from build123d import *

# Parameters (mm, degrees)
CHAFL_N1_SIZE                       = 1.5
CROQUIS3_W                          = 16
CROQUIS3_H                          = 16
CROQUIS3_R                          = 2
SALIENTE_EXTRUIR1_DEPTH             = 2
SALIENTE_EXTRUIR1_DIRECTION_2_REACH = 43.106


with BuildPart() as part:
    # Croquis1 → Revolución1 (revolve)
    with BuildSketch(Plane.XY, mode=Mode.PRIVATE) as revoluci_n1_sk:
        Polygon((0, 9.55), (24, 9.55), (37.076983597, 2), (37.076983597, 5.464101615), (24.803847577, 12.55), (0, 12.55), align=None)
    revolve(revoluci_n1_sk.sketch.rotate(Axis((0, 0, 0), (1, 0, 0)), 180), axis=Axis((0, 0, 0), (1, 0, 0)))

    # Chaflán1
    chafl_n1_edges = [part.edges().sort_by_distance(p)[0] for p in [
        (0, 9.55, 0),
    ]]
    chamfer(chafl_n1_edges, length=CHAFL_N1_SIZE)

    # Croquis3 → Saliente-Extruir1 (add)
    with BuildSketch(Plane(origin=(37.076983597, 0, 0), x_dir=(0, 0, -1), z_dir=(1, 0, 0))):
        Rectangle(CROQUIS3_W, CROQUIS3_H)
        with Locations(Location((0, 0, 0), (0, 0, 270))):
            Circle(CROQUIS3_R, mode=Mode.SUBTRACT)
    extrude(amount=SALIENTE_EXTRUIR1_DEPTH)

    # Croquis3 → Saliente-Extruir1 direction 2 (add, up to next)
    with BuildSketch(Plane(origin=(37.076983597, 0, 0), x_dir=(0, 0, -1), z_dir=(1, 0, 0)), mode=Mode.PRIVATE) as saliente_extruir1_direction_2_sk1:
        Rectangle(CROQUIS3_W, CROQUIS3_H)
        with Locations(Location((0, 0, 0), (0, 0, 270))):
            Circle(CROQUIS3_R, mode=Mode.SUBTRACT)
    saliente_extruir1_direction_2_tool1 = extrude(saliente_extruir1_direction_2_sk1.sketch, amount=-SALIENTE_EXTRUIR1_DIRECTION_2_REACH, mode=Mode.PRIVATE) - part.part
    add(saliente_extruir1_direction_2_tool1.solids().sort_by_distance((37.076984, -7.773726, 0))[0])


solid = part.part
Geometry check sheet. Reference: the model listing, model coordinates, mm. Give positions to 0.01 mm unless a question says otherwise; leave off trailing zeros. Order: outer loops, then holes, each group sorted by start corner. A loop starts at its lowest first (then second) coordinate and runs counter-clockwise, first axis right, second up. Notation, with made-up numbers: (86.5, 11) - (127.5, 11) arc R22 ccw to (127.5, 41) - close; hole circle Ø2 at (-20, 30.25). An arc over 180 degrees is marked (long way). Answer as a JSON object with one key per item and string values.
(1) Draft check along Y on faces 1 (the cylindrical face through (38, 0, 2)), 2 (the flat face through (34, -8, 0)), 3 (the cylindrical face through (12.91, 7.58, 5.81)), 4 (the conical face through (31.316, -8.12, 3.367)). Enter one of: released by +Y, released by -Y, zero draft, split by the parting line, or undercut.
Report:
{"face 1": "undercut", "face 2": "released by -Y", "face 3": "undercut", "face 4": "split by the parting line"}
(2) Material ranges on line 1 (Z direction, x = 11.25, y = 0); line 2 (Z direction, x = 38.4, y = 0); line 3 (Y direction, x = 14.5, z = 6.25), recorded low to high.
Report:
{"line 1": "-12.55 to -9.55, 9.55 to 12.55", "line 2": "-8 to -2, 2 to 8", "line 3": "-10.88 to -7.22, 7.22 to 10.88"}
(3) Depth check by flat-ended pin: pin 1 Ø4 at (x, y) = (23.5, 6) entering from +Z; pin 2 Ø12 at (x, z) = (9.5, -10) entering from +Y; pin 3 Ø3.5 at (x, y) = (32, 2.5) entering from -Z. Enter the tip coordinate at first touch or a pass-through.
Report:
{"pin 1": "z = 11.9", "pin 2": "y = 11.9", "pin 3": "z = -9.15"}
(4) Cross-section at C-C (x = 29.5). Record the cut outline in (y, z).
Report:
{"outline": "(-8, -8) - (-5.73, -8) arc R9.84 ccw to (5.73, -8) - (8, -8) - (8, -5.73) arc R9.84 ccw to (8, 5.73) - (8, 8) - (5.73, 8) arc R9.84 ccw to (-5.73, 8) - (-8, 8) - (-8, 5.73) arc R9.84 ccw to (-8, -5.73) - close; hole circle Ø12.75 at (0, 0)"}
(5) Cross-section at A-A (z = 0). Record the cut outline in (x, y), then the cut area to 3 significant figures.
Report:
{"outline": "(0, -12.55) - (24.8, -12.55) - (32.68, -8) - (39.08, -8) - (39.08, -2) - (37.08, -2) - (24, -9.55) - (1.5, -9.55) - (0, -11.05) - close; (0, 11.05) - (1.5, 9.55) - (24, 9.55) - (37.08, 2) - (39.08, 2) - (39.08, 8) - (32.68, 8) - (24.8, 12.55) - (0, 12.55) - close", "area": "267 mm^2"}
(6) Cross-section at D-D (x = 22). Record the cut outline in (y, z).
Report:
{"outline": "circle Ø25.1 at (0, 0); hole circle Ø19.1 at (0, 0)"}
